Here's how the part is built. I have some questions about the finished solid (model axes, mm). Face numbers are marked on the shaded views. A direction names the side the tool comes from. Round coordinates to 2 decimals unless told otherwise and drop trailing zeros. Order: outer loops, then holes, each group sorted by start corner. A loop starts at its lowest first (then second) coordinate and runs counter-clockwise, first axis right, second up. Notation, with made-up numbers: (-14, -5.5) -> (38, -5.5) arc R26 ccw to (38, 27.5) -> close; hole circle Ø8 at (89.5, 65.25). An arc over 180 degrees is marked (long way). Use a Markdown table: item, result. Add a question column.
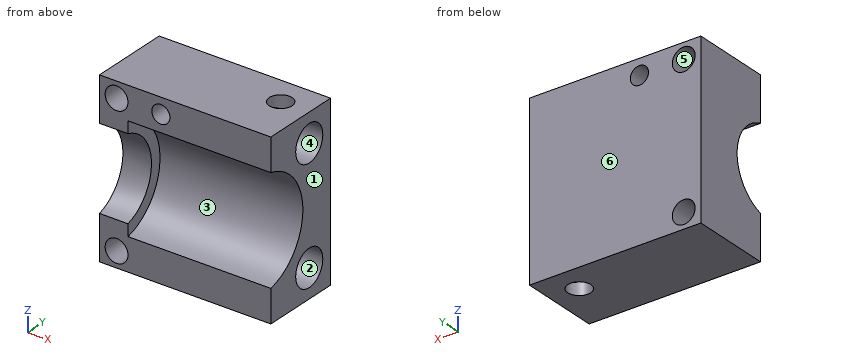
Autodesk Inventor part; units mm, degrees
ref_plane "YZ Plane" through (0, 0, 0) normal (1, 0, 0) x (0, 1, 0)
ref_plane "XZ Plane" through (0, 0, 0) normal (0, 1, 0) x (-1, 0, 0)
ref_plane "XY Plane" through (0, 0, 0) normal (0, 0, 1) x (1, 0, 0)
sketch "Sketch1" plane through (0, 0, 0) normal (0, 0, 1) x (1, 0, 0)
  line L0 (15, -7) -> (-15, -7)
  line L1 (-15, -7) -> (-15, 7)
  line L2 (-15, 7) -> (15, 7)
  line L3 (15, 7) -> (15, -7)
  line L4 (15, -7) -> (-15, 7) construction
  line L5 (-15, -7) -> (15, 7) construction
  point P0 (0, 0)
  dimension "d0" = 30
  dimension "d1" = 14
extrude "Extrusion1" add sketch "Sketch1" along normal blind 30
sketch "Sketch3" plane through (15, -7, 0) normal (1, 0, 0) x (0, 0, -1)
  line L0 (0, 0) -> (-30, 0)
  line L1 (-15, 0) -> (-15, -2)
  arc A0 (-5.7129, 0) -> (-24.2871, 0) centre (-15, -2) ccw
  point P0 (0, 7)
  dimension "d4" = 2
  dimension "d5" = 19
extrude "Extrusion2" cut sketch "Sketch3" against normal blind 25
sketch "Sketch5" plane through (-15, 7, 0) normal (0, 1, 0) x (1, 0, 0)
  line L0 (30, 0) -> (0, 0)
  line L1 (30, -30) -> (0, -30)
  line L2 (0, -30) -> (0, -27.25)
  line L3 (0, 0) -> (0, -30)
  line L4 (0, -27.25) -> (2.75, -27.25)
  circle A0 centre (2.75, -27.25) radius 2
  line L5 (0, 0) -> (0, -2.75)
  line L6 (0, -2.75) -> (2.75, -2.75)
  circle A1 centre (2.75, -2.75) radius 2
  line L7 (2.75, -27.25) -> (10.75, -27.25)
  circle A2 centre (10.75, -27.25) radius 1.5875
  point P0 (15, 0)
  dimension "d11" = 2.75
  dimension "d12" = 2.75
  dimension "d13" = 4
  dimension "d14" = 2.75
  dimension "d15" = 2.75
  dimension "d16" = 4
  dimension "d17" = 8
  dimension "d18" = 3.175
extrude "Extrusion3" cut sketch "Sketch5" against normal blind 100 contours A2
sketch "Sketch6" plane through (-15, 7, 0) normal (0, 1, 0) x (1, 0, 0)
  point P0 (15, 0)
sketch "Sketch7" plane through (15, -7, 0) normal (1, 0, 0) x (0, 0, -1)
  line L0 (0, 14) -> (-30, 14)
  line L1 (-30, 14) -> (-25, 14)
  line L2 (-25, 14) -> (-25, 9)
  line L3 (0, 14) -> (0, 0)
  line L4 (0, 14) -> (-5, 14)
  line L5 (-5, 14) -> (-5, 9)
  circle A0 centre (-25, 9) radius 3.175
  circle A1 centre (-5, 9) radius 3.175
  point P0 (0, 7)
  dimension "d21" = 5
  dimension "d22" = 5
  dimension "d23" = 5
  dimension "d24" = 5
  dimension "d25" = 6.35
  dimension "d26" = 6.35
extrude "Extrusion4" cut sketch "Sketch7" against normal blind 15
move or copy body "Move Body1" bodies to move or copy 1 copy no translate (-20, 0, 0)
move or copy body "Move Body2" bodies to move or copy 1 copy no translate (-5, 0, 0)
sketch "Sketch8" plane through (0, 0, 0) normal (1, 0, 0) x (0, 1, 0)
  point P0 (0, 0)
sketch "Sketch9" plane through (-40, 7, 0) normal (0, 1, 0) x (1, 0, 0)
  line L0 (30, -30) -> (0, -30)
  line L1 (0, -30) -> (0, -27.25)
  line L2 (0, 0) -> (0, -30)
  line L3 (0, -27.25) -> (3, -27.25)
  circle A0 centre (3, -27.25) radius 2
  line L4 (0, 0) -> (0, -2.75)
  line L5 (0, -2.75) -> (3, -2.75)
  circle A1 centre (3, -2.75) radius 2
  point P0 (40, 0)
  dimension "d35" = 2.75
  dimension "d36" = 3
  dimension "d37" = 4
  dimension "d38" = 2.75
  dimension "d39" = 4
  dimension "d40" = 3
extrude "Extrusion5" cut sketch "Sketch9" against normal blind 14
sketch "Sketch14" plane through (-40, 7, 30) normal (0, 0, 1) x (1, 0, 0)
  line L0 (30, 0) -> (0, 0)
  line L1 (30, 0) -> (25, 0)
  line L2 (25, 0) -> (25, -5)
  circle A0 centre (25, -5) radius 2
  point P0 (40, -7)
  dimension "d47" = 5
  dimension "d48" = 5
  dimension "d49" = 4
extrude "Extrusion6" cut sketch "Sketch14" against normal blind 3
sketch "Sketch15" plane through (-10, 7, 0) normal (0, 0, -1) x (-1, 0, 0)
  line L0 (0, -14) -> (0, 0)
  line L1 (0, 0) -> (5, 0)
  line L2 (0, 0) -> (30, 0)
  line L3 (5, 0) -> (5, -5)
  circle A0 centre (5, -5) radius 2
  point P0 (-10, -7)
  dimension "d52" = 5
  dimension "d53" = 5
  dimension "d54" = 4
extrude "Extrusion7" cut sketch "Sketch15" against normal blind 4
thread "Thread3"
thread "Thread4"
sketch "Sketch16" plane through (-40, -7, 0) normal (-1, 0, 0) x (0, 0, 1)
  line L0 (0, 14) -> (30, 14)
  line L1 (0, 14) -> (15, 14)
  line L2 (15, 14) -> (15, -2)
  circle A0 centre (15, -2) radius 7.5
  point P0 (0, 7)
  dimension "d61" = 16
  dimension "d62" = 15
extrude "Extrusion8" cut sketch "Sketch16" against normal blind 15
move or copy body "Move Body3" bodies to move or copy 1 copy no translate (25, 0, 0)
move or copy body "Move Body4" bodies to move or copy 1 copy no translate (10, 0, -15)
move or copy body "Move Body5" bodies to move or copy 1 copy no translate (-10, 0, 0)
sketch "Sketch17" plane through (15, -7, -15) normal (1, 0, 0) x (0, 0, -1)
  point P0 (-15, 7)
equation "\"d55\" = d54"
properties part number "Rb oven housing top-back" material "Copper"
(1) I want a section at B-B on x = -12. List the corners of the cut face in (y, z) for me, and give its area (3 significant figures).
(2) On a 3-axis mill with a long thin cutter (end or side, diameter ignored), from which of +Z, -Z, +X, -X, +Y, -Y can I reach the whole of each face in a straight line? I mean the marked faces 1, 2 and 3. Say none if no direction works.
(3) Please list where these lines run through material, in increasing order: probe 1 along X at (y, z) = (3.5, 12.25); probe 2 along Z at (x, y) = (4.5, 2) (3 decimals); probe 3 along X at (y, z) = (-1, 12.25). Write a range as from..to.
(4) I'm going to push flat-ended pins straight in: P1, Ø6.5, axis at x = 10, y = 2, coming from the +Z side; P2, Ø1.9, axis at y = 2, z = 10, coming from the +X side; P3, Ø4, axis at x = 0, z = -0.5, coming from the -Y side; P4, Ø2.5, axis at x = -12, z = 12.25, coming from the -Y side. Where does each tip first touch, or does it pass through?
(5) I want a section at D-D on x = -4.25. List the corners of the cut face in (y, z) for me, and give its area (3 significant figures).
(6) If we mould it in two halves opening along Y, with no side actions, what happens to the marked faces 4, 5 and 6? For each: pulls with the +Y half, pulls with the -Y half, needs draft (parallel to the pull), parting line crosses it, or undercut.
(7) I want a section at A-A on y = 2. State how many separate pieces and enclosed holes the cut face has, and give its area (3 significant figures).
Output:
| question | item | result |
|---|---|---|
| 1 | outline | (-7, -15) -> (7, -15) -> (7, -14.25) -> (-7, -14.25) -> close; (-7, -10.25) -> (7, -10.25) -> (7, 10.25) -> (-7, 10.25) -> (-7, 7.23) arc R7.5 cw to (-7, -7.23) -> close; (-7, 14.25) -> (7, 14.25) -> (7, 15) -> (-7, 15) -> close |
| 1 | area | 249 mm² |
| 2 | face 1 | +Z, -Z, +X, +Y, -Y |
| 2 | face 2 | +X |
| 2 | face 3 | +X, -Y |
| 3 | probe 1 | -15..-14, -10..-5.84, -2.66..0 |
| 3 | probe 2 | -15..-13.175, -6.825..6.825, 13.175..15 |
| 3 | probe 3 | -15..-14, -10..-5.84, -2.66..15 |
| 4 | P1 | z = 15 |
| 4 | P2 | x = 0 |
| 4 | P3 | y = 0.17 |
| 4 | P4 | through |
| 5 | outline | (-7, -15) -> (7, -15) -> (7, 10.66) -> (-7, 10.66) -> (-7, 9.29) arc R9.5 cw to (-7, -9.29) -> close; (-7, 13.84) -> (7, 13.84) -> (7, 15) -> (-7, 15) -> close |
| 5 | area | 272 mm² |
| 6 | face 4 | undercut |
| 6 | face 5 | needs draft |
| 6 | face 6 | pulls with the +Y half |
| 7 | separate pieces | 3 |
| 7 | enclosed holes | 3 |
| 7 | area | 662 mm² |
